CAD build for the part. Positions are in the model's coordinates, mm. A direction names the side the tool comes from. Coordinates: 2 decimals unless noted, no trailing zeros. Loops run counter-clockwise (first coordinate to the right, second up) from the corner with the lowest first, then second, coordinate; pieces in that order, holes last. Notation, with made-up numbers: (-37.5, -27.5) -> (-27.5, -27.5) arc R17 ccw to (-27.5, -9.5) -> close; hole circle Ø4 at (-20, -7.5). An arc over 180 degrees is marked (long way). Write each question's results on one line, items separated by ' | '.
from build123d import *

# Parameters (mm, degrees)
F1_W     = 20
F1_H     = 40
F1_R     = 2.65
F1_R_2   = 5
F2_DEPTH = 8
F3_R     = 4.3
F4_DEPTH = 4
F5_R     = 2.5
F6_W     = 0.25
F6_H     = 6
F7_DEPTH = 1


with BuildPart() as f2:
    # F1 (on Top) → F2 (new body)
    with BuildSketch(Plane.XY):
        Rectangle(F1_W, F1_H)
        with Locations((0, -14)):
            Circle(F1_R, mode=Mode.SUBTRACT)
        Circle(F1_R_2, mode=Mode.SUBTRACT)
        with Locations((0, 14)):
            Circle(F1_R, mode=Mode.SUBTRACT)
    extrude(amount=F2_DEPTH)

    # F3 (on face) → F4 (cut)
    with BuildSketch(Plane.XY.offset(8)):
        with Locations((0, 14)):
            Circle(F3_R)
        with Locations((0, -14)):
            Circle(F3_R)
    extrude(amount=-F4_DEPTH, mode=Mode.SUBTRACT)

    # F5
    f5_edges = [f2.edges().sort_by_distance(p)[0] for p in [
        (10, -20, 4),
        (-10, -20, 4),
        (10, 20, 4),
        (-10, 20, 4),
    ]]
    fillet(f5_edges, radius=F5_R)

    # F6 (on face) → F7 (cut)
    with BuildSketch(Plane.YZ.offset(10)):
        with Locations((0.125, 3)):
            Rectangle(F6_W, F6_H)
        with Locations((-0.125, 3)):
            Rectangle(F6_W, F6_H)
    extrude(amount=-F7_DEPTH, mode=Mode.SUBTRACT)


solid = f2.part
1) Which spindle directions (+Z, -Z, +X, -X, +Y, -Y) get a long thin tool onto all of the face, cutting with end or side? Do faces 4 (the cylindrical face through (-9.287, 19.248, 4.056)), 5 (the cylindrical face through (-0.56, 18.263, 6.028)), 6 (the flat face through (9.5, -0.25, 3)). Say none if no direction does.
Outcome:
face 4: +Z, -Z, -X, +Y | face 5: +Z | face 6: -Z, +X
2) Slice it at B-B (y = 14). Write the cut outline in (x, z).
Outcome:
outline: (-10, 0) -> (-2.65, 0) -> (-2.65, 4) -> (-4.3, 4) -> (-4.3, 8) -> (-10, 8) -> close; (2.65, 0) -> (10, 0) -> (10, 8) -> (4.3, 8) -> (4.3, 4) -> (2.65, 4) -> close
3) Two-plate mould, pull along X, no slides. Class faces 1 (the flat face through (-2, 12, 4)), 2 (the flat face through (10, 0, 7)), 3 (the flat face through (9.5, 0.25, 3)): pulls with the +X half, pulls with the -X half, needs draft (parallel to the pull), parting line crosses it, or undercut.
Outcome:
face 1: undercut | face 2: pulls with the +X half | face 3: needs draft
4) Slice it at C-C (x = 0). Write the cut outline in (y, z).
Outcome:
outline: (-20, 0) -> (-16.65, 0) -> (-16.65, 4) -> (-18.3, 4) -> (-18.3, 8) -> (-20, 8) -> close; (-11.35, 0) -> (-5, 0) -> (-5, 8) -> (-9.7, 8) -> (-9.7, 4) -> (-11.35, 4) -> close; (5, 0) -> (11.35, 0) -> (11.35, 4) -> (9.7, 4) -> (9.7, 8) -> (5, 8) -> close; (16.65, 0) -> (20, 0) -> (20, 8) -> (18.3, 8) -> (18.3, 4) -> (16.65, 4) -> close
5) Pin check, flat tips, straight feed: pin 1 (7 mm diameter, centred on x = 0, y = -14, fed in from +Z); pin 2 (0.5 mm diameter, centred on x = 9.5, z = 3, fed in from +Y); pin 3 (1.1 mm diameter, centred on x = 9.5, z = 2, fed in from -Y). Stop position of each tip, or through.
Outcome:
pin 1: stops at z = 4 | pin 2: stops at y = 19.29 | pin 3: stops at y = -19.54
6) Drill centre lines: L1, parallel to Y at x = 0, z = 2.8; L2, parallel to Y at x = 0, z = 5.95; L3, parallel to X at y = -14, z = 1.35. Where is each one in solid material? Low to high. Write a range as from..to.
Outcome:
L1: y = -20..-16.65, -11.35..-5, 5..11.35, 16.65..20 | L2: y = -20..-18.3, -9.7..-5, 5..9.7, 18.3..20 | L3: x = -10..-2.65, 2.65..10
7) Slice it at D-D (y = -15). Write the cut outline in (x, z).
Outcome:
outline: (-10, 0) -> (-2.45, 0) -> (-2.45, 4) -> (-4.18, 4) -> (-4.18, 8) -> (-10, 8) -> close; (2.45, 0) -> (10, 0) -> (10, 8) -> (4.18, 8) -> (4.18, 4) -> (2.45, 4) -> close
8) Slice it at A-A (z = 7.25). Write the cut outline in (x, y).
Outcome:
outline: (-10, -17.5) arc R2.5 ccw to (-7.5, -20) -> (7.5, -20) arc R2.5 ccw to (10, -17.5) -> (10, 17.5) arc R2.5 ccw to (7.5, 20) -> (-7.5, 20) arc R2.5 ccw to (-10, 17.5) -> close; hole circle Ø10 at (0, 0); hole circle Ø8.6 at (0, -14); hole circle Ø8.6 at (0, 14)
